from build123d import *


with BuildPart() as part:
    # Çizim1 → Döndür1 (revolve)
    with BuildSketch(Plane.XY, mode=Mode.PRIVATE) as d_nd_r1_sk:
        with BuildLine():
            Line((-62.624886052, 17.432352941), (-62.624886052, 7.632352941))
            ThreePointArc((-62.624886052, 7.632352941), (-62.566307408, 7.490931585), (-62.424886052, 7.432352941))
            Line((-62.424886052, 7.432352941), (-52.843147752, 7.432352941))
            ThreePointArc((-52.843147752, 7.432352941), (-52.695692285, 7.367470983), (-52.643908812, 7.214921793))
            Line((-52.643908812, 7.214921793), (-54.319118015, -11.932807009))
            ThreePointArc((-54.319118015, -11.932807009), (-54.319118015, -14.547479292), (-53.865084938, -17.122428827))
            Line((-53.865084938, -17.122428827), (-49.890893837, -31.954311932))
            Line((-49.890893837, -31.954311932), (-50.373856751, -32.083721455))
            Line((-50.373856751, -32.083721455), (-54.370866241, -17.166678957))
            ThreePointArc((-54.370866241, -17.166678957), (-54.824899318, -14.591729422), (-54.824899318, -11.977057139))
            Line((-54.824899318, -11.977057139), (-53.189563063, 6.714921793))
            ThreePointArc((-53.189563063, 6.714921793), (-53.241346535, 6.867470983), (-53.388802002, 6.932352941))
            Line((-53.388802002, 6.932352941), (-62.924886052, 6.932352941))
            ThreePointArc((-62.924886052, 6.932352941), (-63.066307408, 6.990931585), (-63.124886052, 7.132352941))
            Line((-63.124886052, 7.132352941), (-63.124886052, 17.432352941))
            Line((-63.124886052, 17.432352941), (-62.624886052, 17.432352941))
        make_face()
    revolve(d_nd_r1_sk.sketch.rotate(Axis((0, 0, 0), (0, 1, 0)), 270), axis=Axis((0, 0, 0), (0, 1, 0)))


solid = part.part
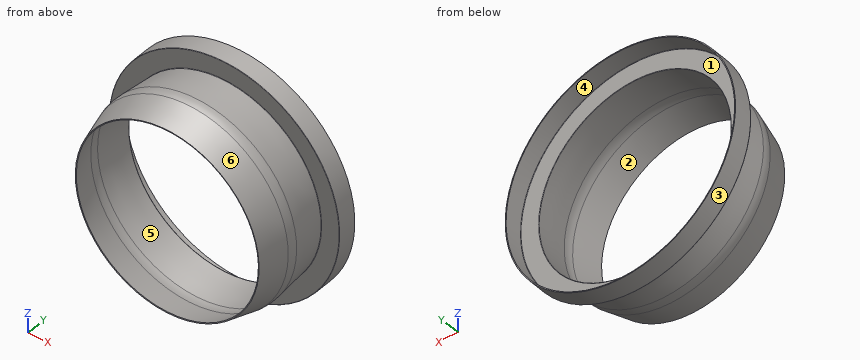
Design review of the part built by this model. Coordinates are the model's own, in mm. Face numbers are marked on the shaded views. A direction names the side the tool comes from. Coordinates: 2 decimals unless noted, no trailing zeros. Order: outer loops, then holes, each group sorted by start corner. A loop starts at its lowest first (then second) coordinate and runs counter-clockwise, first axis right, second up.
Item 1: Take a section at B-B, the plane y = 14.5. Write out the cut boundary in (x, z), then the cut area to 3 significant figures.
Item 2: For line 1 (X direction, y = 12, z = 0); line 2 (X direction, y = -14.5, z = -49); line 3 (Y direction, x = -57, z = -8), list the stretches that pass through material, from the lowest coordinate up.
Item 3: For the marked faces 4, 5 and 6, list the 3-axis set-ups (+Z, -Z, +X, -X, +Y, -Y) from which the entire face can be reached by the end or side of a thin tool; tool diameter is ignored.
Item 4: For pin 1 Ø8 at (x, y) = (24, -3) entering from +Z; pin 2 Ø2 at (x, y) = (-33, -15.5) entering from +Z; pin 3 Ø5 at (x, y) = (-34.5, -19) entering from -Z, all flat-tipped, find the tip position at first contact; note any pin that passes through.
Item 5: Take a section at D-D, the plane y = -20. Write out the cut boundary in (x, z), then the cut area to 3 significant figures.
Item 6: The part is to be moulded in two halves that separate along Y. For the marked faces 1, 2 and 3, say which applies: pulls with the +Y half, pulls with the -Y half, needs draft (parallel to the pull), parting line crosses it, or undercut.
The answers:
1. outline: circle Ø126.25 at (0, 0); hole circle Ø125.25 at (0, 0)
1. area: 198 mm2
2. line 1: x = -63.12 to -62.62, 62.62 to 63.12
2. line 2: x = -24.61 to -23.45, 23.45 to 24.61
2. line 3: y = 6.93 to 7.43
3. face 4: +Y
3. face 5: none
3. face 6: -Y
4. pin 1: stops at z = 50.25
4. pin 2: stops at z = 44.41
4. pin 3: stops at z = -43.53
5. outline: circle Ø107.22 at (0, 0); hole circle Ø106.19 at (0, 0)
5. area: 174 mm2
6. face 1: pulls with the +Y half
6. face 2: undercut
6. face 3: needs draft
